The figure shows three views and two pictorial views of one solid part (mm, origin at its lowest corner). Answer the questions. A direction names the side the tool comes from. Give positions to 0.01 mm unless a question says otherwise; leave off trailing zeros. Loops run counter-clockwise (first coordinate to the right, second up) from the corner with the lowest first, then second, coordinate; pieces in that order, holes last. Notation, with made-up numbers: (11, -22.5) - (40, -22.5) arc R23 ccw to (40, 3.5) - close; hole circle Ø4 at (24.25, -2.5). An arc over 180 degrees is marked (long way). Use a Markdown table: item, result. Add a question column.
Item 1: For a pull along X with two mould halves and no side action, classify the marked faces 4, 5 and 6 as +X half, -X half, draft (parallel to the pull), parting line (faces both ways), or undercut.
Item 2: A cutting plane is placed at A-A (x = 9.85). Determine the outline of the cut face in (y, z).
Item 3: Which of the six approach directions +Z, -Z, +X, -X, +Y, -Y give full straight-line access (tool end or side, diameter ignored) to the marked faces 1, 2 and 3?
Item 4: Each of these flat-tipped pins is pushed along its axis until it touches: P1, Ø1.5, axis at x = 13, z = 14, coming from the +Y side; P2, Ø6, axis at x = 11, z = 1.5, coming from the +Y side; P3, Ø5, axis at x = 12, y = 9, coming from the -Z side; P4, Ø6, axis at y = 6, z = 2, coming from the -X side. Where does it stop, or does it pass through?
Item 5: A cutting plane is placed at B-B (z = 12.5). Determine the outline of the cut face in (x, y), plus the area to 3 significant figures.
Item 6: A cutting plane is placed at C-C (z = 1.75). Determine the outline of the cut face in (x, y).
Item 7: Consider probe 1 along Y at (x, z) = (9.85, 6.7); probe 2 along Y at (x, z) = (9.85, 1.2). Determine where each line is inside the solid, lowest interval first. Write a range as [from, to].
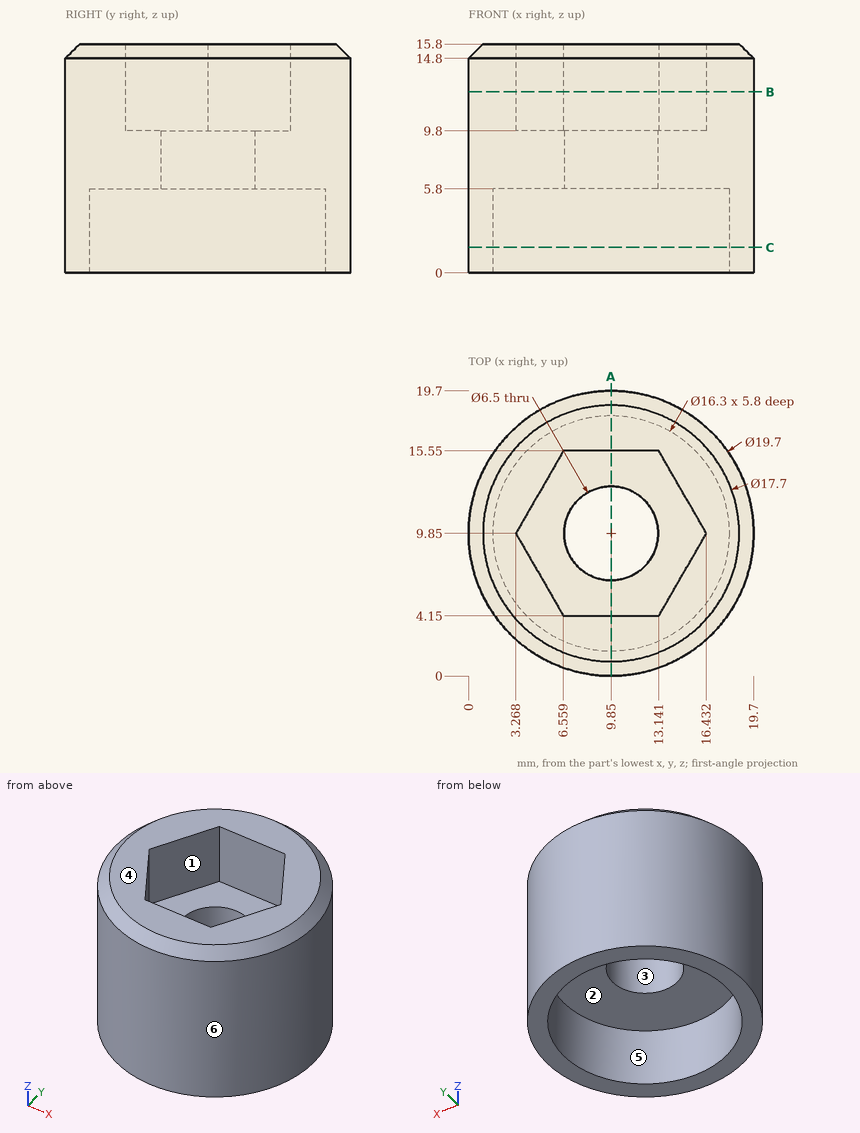
Geometry says:
| question | item | result |
|---|---|---|
| 1 | face 4 | draft |
| 1 | face 5 | undercut |
| 1 | face 6 | parting line |
| 2 | outline | (0, 0) - (1.7, 0) - (1.7, 5.8) - (6.6, 5.8) - (6.6, 9.8) - (4.15, 9.8) - (4.15, 15.8) - (1, 15.8) - (0, 14.8) - close; (13.1, 5.8) - (18, 5.8) - (18, 0) - (19.7, 0) - (19.7, 14.8) - (18.7, 15.8) - (15.55, 15.8) - (15.55, 9.8) - (13.1, 9.8) - close |
| 3 | face 1 | +Z |
| 3 | face 2 | -Z |
| 3 | face 3 | +Z, -Z |
| 4 | P1 | y = 19.4 |
| 4 | P2 | y = 19.7 |
| 4 | P3 | z = 5.8 |
| 4 | P4 | x = 0.04 |
| 5 | outline | circle Ø19.7 at (9.85, 9.85); hole (3.27, 9.85) - (6.56, 4.15) - (13.14, 4.15) - (16.43, 9.85) - (13.14, 15.55) - (6.56, 15.55) - close |
| 5 | area | 192 mm² |
| 6 | outline | circle Ø19.7 at (9.85, 9.85); hole circle Ø16.3 at (9.85, 9.85) |
| 7 | probe 1 | [0, 6.6], [13.1, 19.7] |
| 7 | probe 2 | [0, 1.7], [18, 19.7] |
